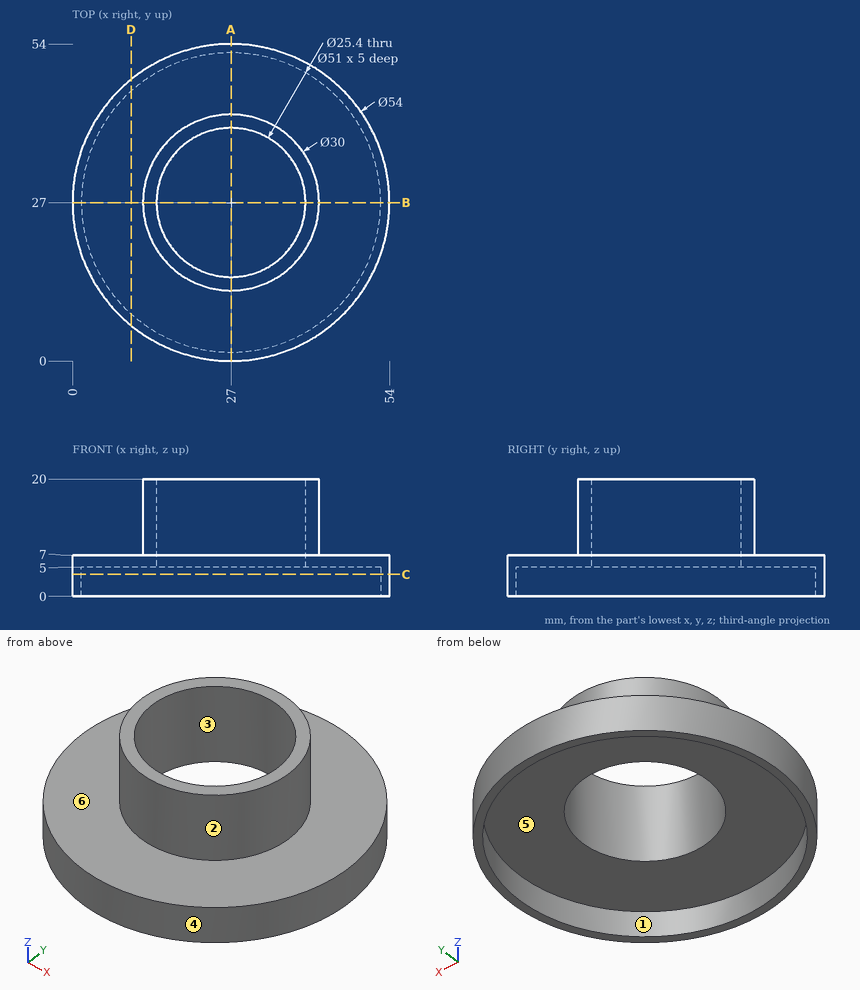
Design review of the part shown in the three views and the two pictorial views. Dimensions are in mm from the part's minimum x, y and z. A direction names the side the tool comes from. Coordinates: 2 decimals unless noted, no trailing zeros. Loops run counter-clockwise (first coordinate to the right, second up) from the corner with the lowest first, then second, coordinate; pieces in that order, holes last.
Q1. For pin 1 (4 mm diameter, centred on x = 48, y = 34.5, fed in from +Z); pin 2 (4 mm diameter, centred on y = 28.5, z = 10, fed in from -X); pin 3 (1.5 mm diameter, centred on x = 48, z = 7.5, fed in from +Y); pin 4 (23 mm diameter, centred on x = 27, y = 27, fed in from -Z), all flat-tipped, find the tip position at first contact; note any pin that passes through.
Reported:
pin 1: stops at z = 7
pin 2: stops at x = 12
pin 3: stops at y = 44.64
pin 4: passes through
Q2. We need section D-D on x = 10. State the section outline as (y, z) points.
Reported:
outline: (6.02, 0) - (7.99, 0) - (7.99, 5) - (46.01, 5) - (46.01, 0) - (47.98, 0) - (47.98, 7) - (6.02, 7) - close
Q3. The part is to be moulded in two halves that separate along Y. For the marked faces 4, 5 and 6, say which applies: +Y half, -Y half, draft (parallel to the pull), parting line (faces both ways), or undercut.
Reported:
face 4: parting line
face 5: undercut
face 6: draft
Q4. We need section A-A on x = 27. State the section outline as (y, z) points.
Reported:
outline: (0, 0) - (1.5, 0) - (1.5, 5) - (14.3, 5) - (14.3, 20) - (12, 20) - (12, 7) - (0, 7) - close; (39.7, 5) - (52.5, 5) - (52.5, 0) - (54, 0) - (54, 7) - (42, 7) - (42, 20) - (39.7, 20) - close
Q5. Tool access review of the marked faces 1, 2 and 3: name each direction out of +Z, -Z, +X, -X, +Y, -Y from which nothing blocks a thin tool from reaching the whole face with its end or side.
Reported:
face 1: -Z
face 2: +Z
face 3: +Z, -Z
Q6. To check wall thickness, follow line 1 (Y direction, x = 27, z = 2.85); line 2 (Y direction, x = 27, z = 11.25); line 3 (Z direction, x = 15, y = 5). State the ranges of each line that lie inside material, in increasing order.
Reported:
line 1: y = 0 to 1.5, 52.5 to 54
line 2: y = 12 to 14.3, 39.7 to 42
line 3: z = 5 to 7
Q7. We need section C-C on z = 3.75. State the section outline as (x, y) points, and give its area (3 significant figures).
Reported:
outline: circle Ø54 at (27, 27); hole circle Ø51 at (27, 27)
area: 247 mm2
